The model under review builds one solid part; all positions refer to its coordinate system, in mm. Coordinates: 2 decimals unless noted, no trailing zeros. Order: outer loops, then holes, each group sorted by start corner. A loop starts at its lowest first (then second) coordinate and runs counter-clockwise, first axis right, second up. Notation, with made-up numbers: (68.5, -30.5) - (72.5, -30.5) arc R30 ccw to (72.5, 5.5) - close; hole circle Ø8 at (-0.5, -25.5). An arc over 180 degrees is marked (long way). Answer in a Markdown table with one row per item.
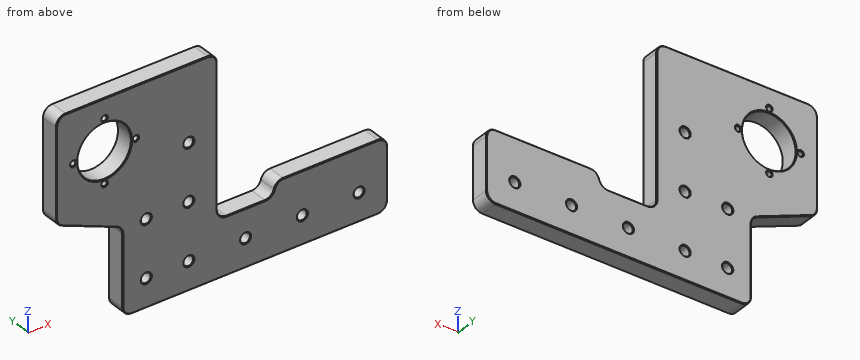
```python
from build123d import *

# Parameters (mm, degrees)
F0_R     = 3.2639
F0_R_2   = 1.7018
F0_R_3   = 17.9959
F1_DEPTH = 12.7
F2_W     = 107.95
F2_H     = 19.2481796932
F3_DEPTH = 25.4
F4_F1_R  = 6.35
F4_F2_R  = 6.35
F5_R     = 6.35
F6_SIZE  = 0.508


with BuildPart() as f1:
    # F0 (on Front) → F1 (new body)
    with BuildSketch(Plane.XZ):
        Polygon((-126.667948618, -98.7711842824), (95.582051382, -98.4536048876), (95.582051382, -60.3536048876), (95.582051382, -50.8286048876), (19.382051382, -50.8286048876), (19.382051382, -60.3536048876), (-18.717948618, -60.3536048876), (-18.717948618, 66.3288157176), (-126.667948618, 66.3288157176), align=None)
        with Locations((-66.3308787224, -79.5945032566)):
            Circle(F0_R, mode=Mode.SUBTRACT)
        with Locations((-37.7828981478, -79.5941544378)):
            Circle(F0_R, mode=Mode.SUBTRACT)
        with Locations((-66.3853614397, -41.4661356021)):
            Circle(F0_R, mode=Mode.SUBTRACT)
        with Locations((-37.7829381848, -41.4661356021)):
            Circle(F0_R, mode=Mode.SUBTRACT)
        with Locations((0.3171018521, -79.5941544378)):
            Circle(F0_R, mode=Mode.SUBTRACT)
        with Locations((38.4171018521, -79.5941544378)):
            Circle(F0_R, mode=Mode.SUBTRACT)
        with Locations((76.5171018521, -79.5941544378)):
            Circle(F0_R, mode=Mode.SUBTRACT)
        with Locations((-117.8233242227, -10.5161073038)):
            Circle(F0_R_2, mode=Mode.SUBTRACT)
        with Locations((-94.3283242227, -8.0269073038)):
            Circle(F0_R_2, mode=Mode.SUBTRACT)
        with Locations((-115.3341242227, 12.9788926962)):
            Circle(F0_R_2, mode=Mode.SUBTRACT)
        with Locations((-94.3283242227, 12.9788926962)):
            Circle(F0_R_3, mode=Mode.SUBTRACT)
        with Locations((-73.3225242227, 12.9788926962)):
            Circle(F0_R_2, mode=Mode.SUBTRACT)
        with Locations((-70.8333242227, -10.5161073038)):
            Circle(F0_R_2, mode=Mode.SUBTRACT)
        with Locations((-37.7829381848, -3.3661356021)):
            Circle(F0_R, mode=Mode.SUBTRACT)
        with Locations((-117.8233242227, 36.4738926962)):
            Circle(F0_R_2, mode=Mode.SUBTRACT)
        with Locations((-94.3283242227, 33.9846926962)):
            Circle(F0_R_2, mode=Mode.SUBTRACT)
        with Locations((-70.8333242227, 36.4738926962)):
            Circle(F0_R_2, mode=Mode.SUBTRACT)
        with Locations((-117.8233242227, 36.4738926962)):
            Circle(F0_R_2)
        with Locations((-70.8333242227, 36.4738926962)):
            Circle(F0_R_2)
        with Locations((-70.8333242227, -10.5161073038)):
            Circle(F0_R_2)
        with Locations((-117.8233242227, -10.5161073038)):
            Circle(F0_R_2)
    extrude(amount=F1_DEPTH)

    # F2 (on face) → F3 (cut)
    with BuildSketch(Plane.XZ.offset(12.7)):
        Polygon((-82.2601616383, -40.8437248283), (-126.667948618, -22.6552803069), (-126.667948618, -98.7711842824), (-82.2601616383, -98.7077287228), align=None)
        with Locations((-72.692948618, 56.7047258711)):
            Rectangle(F2_W, F2_H)
    extrude(amount=-F3_DEPTH, mode=Mode.SUBTRACT)

    # F4: fillet of radius 6.35 on 9 edges, made by hand

    # F4_f1
    f4_f1_edges = [f1.edges().sort_by_distance(p)[0] for p in [
        (-82.2601616383, -6.35, -40.8437248283),
        (-18.717948618, -6.35, -60.3536048876),
    ]]
    fillet(f4_f1_edges, radius=F4_F1_R)

    # F4_f2
    f4_f2_edges = [f1.edges().sort_by_distance(p)[0] for p in [
        (-126.667948618, -6.35, 47.0806360245),
        (-126.667948618, -6.35, -22.6552803069),
        (-18.717948618, -6.35, 47.0806360245),
        (-82.2601616383, -6.35, -98.7077287228),
        (95.582051382, -6.35, -98.4536048876),
        (95.582051382, -6.35, -50.8286048876),
        (19.382051382, -6.35, -50.8286048876),
    ]]
    fillet(f4_f2_edges, radius=F4_F2_R)

    # F5
    f5_edges = [f1.edges().sort_by_distance(p)[0] for p in [
        (19.382051, -6.35, -60.353605),
    ]]
    fillet(f5_edges, radius=F5_R)

    # F6
    f6_edges = [f1.edges().sort_by_distance(p)[0] for p in [
        (21.843486, -12.7, -52.158489),
        (17.323894, -12.7, -59.023721),
        (57.482051, -12.7, -50.828605),
        (0.53369, -12.7, -60.353605),
        (93.722179, -12.7, -52.688477),
        (-16.858077, -12.7, -58.493733),
        (95.582051, -12.7, -74.645638),
        (-18.717949, -12.7, -6.636484),
        (93.725386, -12.7, -96.599591),
        (-20.577821, -12.7, 45.220764),
        (6.670019, -12.7, -98.580654),
        (-72.692949, -12.7, 47.080636),
        (-80.397081, -12.7, -96.841983),
        (-124.808077, -12.7, 45.220764),
        (-82.260162, -12.7, -68.726767),
        (-126.667949, -12.7, 11.168258),
        (-83.337331, -12.7, -41.566558),
        (-125.590779, -12.7, -21.932447),
        (-104.464055, -12.7, -31.749503),
        (-69.594779, -12.7, -79.594503),
        (-41.046798, -12.7, -79.594154),
        (-69.649261, -12.7, -41.466136),
        (-41.046838, -12.7, -41.466136),
        (-2.946798, -12.7, -79.594154),
        (35.153202, -12.7, -79.594154),
        (73.253202, -12.7, -79.594154),
        (-96.030124, -12.7, -8.026907),
        (-41.046838, -12.7, -3.366136),
        (-117.035924, -12.7, 12.978893),
        (-112.324224, -12.7, 12.978893),
        (-75.024324, -12.7, 12.978893),
        (-96.030124, -12.7, 33.984693),
        (21.843486, 0, -52.158489),
        (17.323894, 0, -59.023721),
        (57.482051, 0, -50.828605),
        (0.53369, 0, -60.353605),
        (93.722179, 0, -52.688477),
        (-16.858077, 0, -58.493733),
        (95.582051, 0, -74.645638),
        (-18.717949, 0, -6.636484),
        (93.725386, 0, -96.599591),
        (-20.577821, 0, 45.220764),
        (6.670019, 0, -98.580654),
        (-72.692949, 0, 47.080636),
        (-80.397081, 0, -96.841983),
        (-124.808077, 0, 45.220764),
        (-82.260162, 0, -68.726767),
        (-126.667949, 0, 11.168258),
        (-83.337331, 0, -41.566558),
        (-125.590779, 0, -21.932447),
        (-104.464055, 0, -31.749503),
        (-69.594779, 0, -79.594503),
        (-41.046798, 0, -79.594154),
        (-69.649261, 0, -41.466136),
        (-41.046838, 0, -41.466136),
        (-2.946798, 0, -79.594154),
        (35.153202, 0, -79.594154),
        (73.253202, 0, -79.594154),
        (-96.030124, 0, -8.026907),
        (-41.046838, 0, -3.366136),
        (-117.035924, 0, 12.978893),
        (-112.324224, 0, 12.978893),
        (-75.024324, 0, 12.978893),
        (-96.030124, 0, 33.984693),
    ]]
    chamfer(f6_edges, length=F6_SIZE)


solid = f1.part
```
Item 1: We need section C-C, the plane y = -4.75. State how many separate pieces and enclosed holes the cut face has, then the cut area to 3 significant figures.
Check values:
| item | result |
|---|---|
| separate pieces | 1 |
| enclosed holes | 13 |
| area | 16,500 mm^2 |
Item 2: To check wall thickness, follow line 1 (X direction, y = -8, z = -79); line 2 (Z direction, x = -63.5, y = -1.5); line 3 (Z direction, x = -94, y = -11.5). State the ranges of each line that lie inside material, in increasing order. Write a range as from..to.
Check values:
| item | result |
|---|---|
| line 1 | -82.26..-69.54, -63.12..-40.99, -34.57..-2.89, 3.53..35.21, 41.63..73.31, 79.73..95.58 |
| line 2 | -98.68..-81.22, -77.97..-42.99, -39.94..47.08 |
| line 3 | -36.04..-9.7, -6.36..-5.01, 30.97..32.31, 35.65..47.08 |
Item 3: We need section A-A, the plane z = -87. Write out the cut boundary in (x, y), then the cut area to 3 significant figures.
Check values:
| item | result |
|---|---|
| outline | (-82.26, -12.19) - (-81.75, -12.7) - (95.07, -12.7) - (95.58, -12.19) - (95.58, -0.51) - (95.07, 0) - (-81.75, 0) - (-82.26, -0.51) - close |
| area | 2,260 mm^2 |
Item 4: Clearance check with flat-ended pins moving along their axes: pin 1 Ø8 at (x, z) = (-11.5, -46) entering from -Y; pin 2 Ø2 at (x, y) = (-24.5, -1.5) entering from -Z; pin 3 Ø4 at (x, z) = (-73.32, 12.98) entering from -Y; pin 4 Ø4 at (y, z) = (-7, -37) entering from +X. State where each tip first meets the part, or that it passes through.
Check values:
| item | result |
|---|---|
| pin 1 | through |
| pin 2 | z = -98.63 |
| pin 3 | y = -12.49 |
| pin 4 | x = -18.72 |
Item 5: We need section B-B, the plane x = 66. Write out the cut boundary in (y, z), then the cut area to 3 significant figures.
Check values:
| item | result |
|---|---|
| outline | (-12.7, -97.99) - (-12.19, -98.5) - (-0.51, -98.5) - (0, -97.99) - (0, -51.34) - (-0.51, -50.83) - (-12.19, -50.83) - (-12.7, -51.34) - close |
| area | 605 mm^2 |
